Design review of the part built by this model. Coordinates are the model's own, in mm. Face numbers are marked on the shaded views. A direction names the side the tool comes from. Give positions to 0.01 mm unless a question says otherwise; leave off trailing zeros. Order: outer loops, then holes, each group sorted by start corner. A loop starts at its lowest first (then second) coordinate and runs counter-clockwise, first axis right, second up.
```python
from build123d import *

# Parameters (mm, degrees)
TABAN_FLAN_1_DEPTH      = 135
IZIM2_R                 = 3.2
IZIM2_R_2               = 30
KES_EKSTR_ZYON1_DEPTH   = 10
KENAR_FLAN_1_DEPTH      = 135
KENAR_FLAN_1_BEND_DEPTH = 135
IZIM6_W                 = 32
IZIM6_H                 = 40
KES_EKSTR_ZYON2_DEPTH   = 10
RADYUS2_R               = 10
IZIM10_R                = 4.5
KES_EKSTR_ZYON3_DEPTH   = 10
PAH1_SIZE               = 15
RADYUS3_R               = 10


# Sheet-metal steps are written as plain solids
with BuildPart() as part:
    # Çizim1 → Taban-Flanş1 (new body)
    with BuildSketch(Plane.XY):
        with BuildLine():
            Line((0, 0), (0, 42))
            ThreePointArc((0, 42), (2.343145751, 47.656854249), (8, 50))
            Line((8, 50), (120, 50))
            ThreePointArc((120, 50), (125.656854249, 47.656854249), (128, 42))
            Line((128, 42), (128, 0))
            Line((128, 0), (124, 0))
            Line((124, 0), (124, 42))
            ThreePointArc((124, 42), (122.828427125, 44.828427125), (120, 46))
            Line((120, 46), (8, 46))
            ThreePointArc((8, 46), (5.171572875, 44.828427125), (4, 42))
            Line((4, 42), (4, 0))
            Line((4, 0), (0, 0))
        make_face()
    extrude(amount=TABAN_FLAN_1_DEPTH)

    # Çizim2 → Kes-Ekstrüzyon1 (cut)
    with BuildSketch(Plane(origin=(0, 50, 0), x_dir=(1, 0, 0), z_dir=(0, 1, 0))):
        with Locations(Location((63, -21.5, 0), (0, 0, 270))):
            Circle(IZIM2_R)
        with Locations(Location((102.837168574, -44.5, 0), (0, 0, 270))):
            Circle(IZIM2_R)
        with Locations(Location((102.837168574, -90.5, 0), (0, 0, 270))):
            Circle(IZIM2_R)
        with Locations(Location((63, -113.5, 0), (0, 0, 270))):
            Circle(IZIM2_R)
        with Locations(Location((23.162831426, -90.5, 0), (0, 0, 270))):
            Circle(IZIM2_R)
        with Locations(Location((23.162831426, -44.5, 0), (0, 0, 270))):
            Circle(IZIM2_R)
        with Locations(Location((63, -67.5, 0), (0, 0, 270))):
            Circle(IZIM2_R_2)
    extrude(amount=-KES_EKSTR_ZYON1_DEPTH, mode=Mode.SUBTRACT)

    # Kenar-Flanş1 section (across the edge) → Kenar-Flanş1 (add)
    with BuildSketch(Plane(origin=(128, -4, 135), x_dir=(0, 1, 0), z_dir=(0, 0, -1))):
        with BuildLine():
            Line((-4, 4), (-4, 36))
            Line((-4, 36), (0, 36))
            Line((0, 36), (0, 4))
            ThreePointArc((0, 4), (1.171572875, 1.171572875), (4, 0))
            Line((4, 0), (4, -4))
            ThreePointArc((4, -4), (-1.656854249, -1.656854249), (-4, 4))
        make_face()
    extrude(amount=KENAR_FLAN_1_DEPTH)

    # Kenar-Flanş1 section 2 (across the edge) → Kenar-Flanş1 bend (add)
    with BuildSketch(Plane(origin=(0, -4, 0), x_dir=(0, 1, 0), z_dir=(0, 0, 1))):
        with BuildLine():
            Line((-4, 4), (-4, 36))
            Line((-4, 36), (0, 36))
            Line((0, 36), (0, 4))
            ThreePointArc((0, 4), (1.171572875, 1.171572875), (4, 0))
            Line((4, 0), (4, -4))
            ThreePointArc((4, -4), (-1.656854249, -1.656854249), (-4, 4))
        make_face()
    extrude(amount=KENAR_FLAN_1_BEND_DEPTH)

    # Çizim6 → Kes-Ekstrüzyon2 (cut)
    with BuildSketch(Plane(origin=(0, -4, 0), x_dir=(1, 0, 0), z_dir=(0, 1, 0))):
        with Locations((148, -20)):
            Rectangle(IZIM6_W, IZIM6_H)
    extrude(amount=-KES_EKSTR_ZYON2_DEPTH, mode=Mode.SUBTRACT)

    # Radyus2
    radyus2_edges = [part.edges().sort_by_distance(p)[0] for p in [
        (-36, -6, 0),
        (-36, -6, 135),
        (164, -6, 135),
    ]]
    fillet(radyus2_edges, radius=RADYUS2_R)

    # Çizim10 → Kes-Ekstrüzyon3 (cut)
    with BuildSketch(Plane(origin=(0, -4, 0), x_dir=(1, 0, 0), z_dir=(0, 1, 0))):
        with Locations(Location((148, -115, 0), (0, 0, 180))):
            Circle(IZIM10_R)
        with Locations(Location((148, -60, 0), (0, 0, 180))):
            Circle(IZIM10_R)
        with Locations(Location((-20, -115, 0), (0, 0, 180))):
            Circle(IZIM10_R)
        with Locations(Location((-20, -35, 0), (0, 0, 180))):
            Circle(IZIM10_R)
    extrude(amount=-KES_EKSTR_ZYON3_DEPTH, mode=Mode.SUBTRACT)

    # Pah1
    pah1_edges = [part.edges().sort_by_distance(p)[0] for p in [
        (164, -6, 40),
    ]]
    chamfer(pah1_edges, length=PAH1_SIZE)

    # Radyus3
    radyus3_edges = [part.edges().sort_by_distance(p)[0] for p in [
        (164, -6, 55),
        (149, -6, 40),
    ]]
    fillet(radyus3_edges, radius=RADYUS3_R)


solid = part.part
```
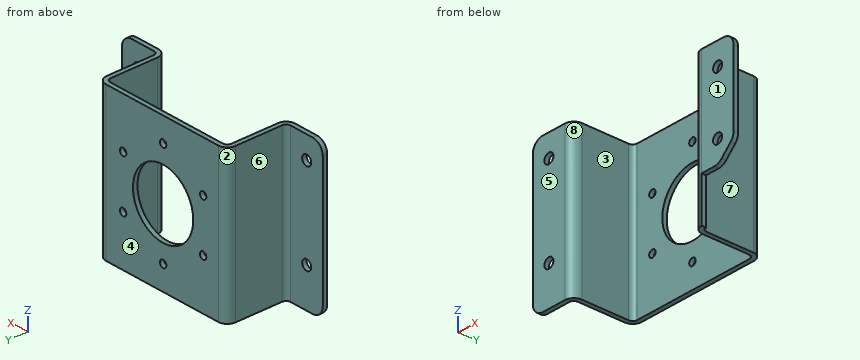
1. For line 1 along Z through (x, y) = (-20, -5.55); line 2 along X through (y, z) = (0.5, 50.5); line 3 along X through (y, z) = (46.8, 90.5), list the stretches that pass through material, from the lowest coordinate up.
Recorded:
line 1: z = 0 to 30.5, 39.5 to 110.5, 119.5 to 135
line 2: x = 0 to 4, 124 to 128
line 3: x = 1.6 to 19.96, 26.36 to 43.74, 82.26 to 99.64, 106.04 to 126.4
2. Take a section at D-D (x = -20). State the section outline as (y, z) points, then the cut area to 3 significant figures.
Recorded:
outline: (-8, 0) - (-4, 0) - (-4, 30.5) - (-8, 30.5) - close; (-8, 39.5) - (-4, 39.5) - (-4, 110.5) - (-8, 110.5) - close; (-8, 119.5) - (-4, 119.5) - (-4, 135) - (-8, 135) - close
area: 468 mm2
3. Take a section at A-A (x = 63). State the section outline as (y, z) points, then the cut area to 3 significant figures.
Recorded:
outline: (46, 0) - (50, 0) - (50, 18.3) - (46, 18.3) - close; (46, 24.7) - (50, 24.7) - (50, 37.5) - (46, 37.5) - close; (46, 97.5) - (50, 97.5) - (50, 110.3) - (46, 110.3) - close; (46, 116.7) - (50, 116.7) - (50, 135) - (46, 135) - close
area: 249 mm2
4. Machinability: for the marked faces 4, 5, 6, 7 and 8, which of the approach directions +Z, -Z, +X, -X, +Y, -Y give a long, thin tool a straight path to every point of the face, cutting with its end or side? Answer none if there is none.
Recorded:
face 4: +Z, -Z, +X, -X, +Y
face 5: +Z, -Z, +X, -X, -Y
face 6: +Z, -Z, -X, +Y
face 7: +Z, -Z, +X, +Y
face 8: +Z, -Z, -Y
5. Take a section at B-B (y = 13.5). State the section outline as (x, z) points, then the cut area to 3 significant figures.
Recorded:
outline: (0, 0) - (4, 0) - (4, 135) - (0, 135) - close; (124, 0) - (128, 0) - (128, 135) - (124, 135) - close
area: 1,080 mm2
6. Take a section at C-C (z = 21.5). State the section outline as (x, y) points, then the cut area to 3 significant figures.
Recorded:
outline: (-36, -8) - (-4, -8) arc R8 ccw to (4, 0) - (4, 42) arc R4 cw to (8, 46) - (59.8, 46) - (59.8, 50) - (8, 50) arc R8 ccw to (0, 42) - (0, 0) arc R4 cw to (-4, -4) - (-36, -4) - close; (66.2, 46) - (120, 46) arc R4 cw to (124, 42) - (124, 0) arc R8 ccw to (132, -8) - (132, -4) arc R4 cw to (128, 0) - (128, 42) arc R8 ccw to (120, 50) - (66.2, 50) - close
area: 1,040 mm2
7. For pin 1 (12.5 mm diameter, centred on y = 27.5, z = 39.5, fed in from +X); pin 2 (21 mm diameter, centred on y = 17, z = 61.5, fed in from -X); pin 3 (16 mm diameter, centred on x = -24, z = 41.5, fed in from +Y); pin 4 (7 mm diameter, centred on x = -20, z = 115, fed in from -Y), all flat-tipped, find the tip position at first contact; note any pin that passes through.
Recorded:
pin 1: stops at x = 128
pin 2: stops at x = 0
pin 3: stops at y = -4
pin 4: passes through
8. Draft analysis for pull direction X (two halves, no side actions). For the marked faces 1, 2 and 3, state which applies: pulls with the +X half, pulls with the -X half, needs draft (parallel to the pull), parting line crosses it, or undercut.
Recorded:
face 1: needs draft
face 2: pulls with the -X half
face 3: undercut
